Verification items for the finished model (mm, model axes). A direction names the side the tool comes from. Give positions to 0.01 mm unless a question says otherwise; leave off trailing zeros. Write each loop counter-clockwise with the first axis right and the second up, starting at its lowest first coordinate (ties: lowest second). Pieces come first, ordered by that corner, then holes.
from build123d import *

# Parameters (mm, degrees)
F1_DEPTH     = 20
F2_T1_DEPTH  = 20
F2_T3_DEPTH  = 35
F3_T1_DEPTH  = 4
F3_T3_DEPTH  = 23.5
F3_T5_DEPTH  = 38.5
F3_T8_ANGLE  = 89.9999999987
F3_T10_ANGLE = 89.9999999987
F3_T12_ANGLE = 89.9999999987
F3_T14_ANGLE = 89.9999999987
F3_T18_ANGLE = 359.64
F3_S19_R     = 5
F3_T20_DEPTH = 6
F3_T24_ANGLE = 359.64
F3_S25_R     = 5
F3_T26_DEPTH = 6
F3_T30_ANGLE = 328.8283154119
F3_S31_R     = 5
F3_T32_DEPTH = 6
F3_T36_ANGLE = 328.8283154119
F3_S37_R     = 5
F3_T38_DEPTH = 6


# Not quite as in the source:
# - a fillet or chamfer that OpenCascade refuses, or shapes differently, is made with other operations: its cross-section is extruded or revolved along the edge and cut away or added


with BuildPart() as f1:
    # F0 (on Right) → F1 (new body)
    with BuildSketch(Plane.YZ):
        Polygon((0, -10.05617938), (0, 24.94382062), (-3, 24.94382062), (-3, -7.05617938), (-13, -7.05617938), (-13, 9.94382062), (-16, 9.94382062), (-16, -10.05617938), align=None)
    extrude(amount=F1_DEPTH)

    # F2: fillet of radius 3 on 5 edges, made by hand

    # F2_s2 → F2_t1 (join)
    with BuildSketch(Plane.YZ):
        with BuildLine():
            ThreePointArc((-10, -7.05617938), (-12.1213203436, -6.1774997235), (-13, -4.05617938))
            Line((-13, -4.05617938), (-13, -7.05617938))
            Line((-13, -7.05617938), (-10, -7.05617938))
        make_face()
        with BuildLine():
            ThreePointArc((-3, -4.05617938), (-3.8786796564, -6.1774997235), (-6, -7.05617938))
            Line((-6, -7.05617938), (-3, -7.05617938))
            Line((-3, -7.05617938), (-3, -4.05617938))
        make_face()
    extrude(amount=F2_T1_DEPTH)

    # F2_s4 → F2_t3 (cut)
    with BuildSketch(Plane.YZ.offset(-7.5)):
        with BuildLine():
            ThreePointArc((0, 24.94382062), (-2.1213203436, 24.0651409636), (-3, 21.94382062))
            Line((-3, 21.94382062), (-3, 24.94382062))
            Line((-3, 24.94382062), (0, 24.94382062))
        make_face()
        with BuildLine():
            ThreePointArc((-13, 6.94382062), (-13.8786796564, 9.0651409636), (-16, 9.94382062))
            Line((-16, 9.94382062), (-13, 9.94382062))
            Line((-13, 9.94382062), (-13, 6.94382062))
        make_face()
        with BuildLine():
            ThreePointArc((-16, 6.94382062), (-15.1213203436, 9.0651409636), (-13, 9.94382062))
            Line((-13, 9.94382062), (-16, 9.94382062))
            Line((-16, 9.94382062), (-16, 6.94382062))
        make_face()
    extrude(amount=F2_T3_DEPTH, mode=Mode.SUBTRACT)

    # F3: fillet of radius 5 on 4 edges, made by hand

    # F3_s2 → F3_t1 (cut)
    with BuildSketch(Plane.XZ.offset(6)):
        with BuildLine():
            ThreePointArc((20, -12.05617938), (18.5355339059, -8.520645474), (15, -7.05617938))
            Line((15, -7.05617938), (20, -7.05617938))
            Line((20, -7.05617938), (20, -12.05617938))
        make_face()
        with BuildLine():
            ThreePointArc((0, -12.05617938), (1.4644660941, -8.520645474), (5, -7.05617938))
            Line((5, -7.05617938), (0, -7.05617938))
            Line((0, -7.05617938), (0, -12.05617938))
        make_face()
    extrude(amount=F3_T1_DEPTH, mode=Mode.SUBTRACT)

    # F3_s4 → F3_t3 (cut)
    with BuildSketch(Plane.XY.offset(-4.05617938)):
        with BuildLine():
            ThreePointArc((20, -18), (18.5355339059, -14.4644660941), (15, -13))
            Line((15, -13), (20, -13))
            Line((20, -13), (20, -18))
        make_face()
        with BuildLine():
            ThreePointArc((0, -18), (1.4644660941, -14.4644660941), (5, -13))
            Line((5, -13), (0, -13))
            Line((0, -13), (0, -18))
        make_face()
    extrude(amount=F3_T3_DEPTH, mode=Mode.SUBTRACT)

    # F3_s6 → F3_t5 (cut)
    with BuildSketch(Plane.XY.offset(-4.05617938)):
        with BuildLine():
            ThreePointArc((20, 2), (18.5355339059, -1.5355339059), (15, -3))
            Line((15, -3), (20, -3))
            Line((20, -3), (20, 2))
        make_face()
        with BuildLine():
            ThreePointArc((0, 2), (1.4644660941, -1.5355339059), (5, -3))
            Line((5, -3), (0, -3))
            Line((0, -3), (0, 2))
        make_face()
    extrude(amount=F3_T5_DEPTH, mode=Mode.SUBTRACT)

    # F3_s7 → F3_t8 (revolve, cut)
    with BuildSketch(Plane.XY.offset(-4.05617938)):
        with BuildLine():
            ThreePointArc((0, 2), (1.4644660941, -1.5355339059), (5, -3))
            Line((5, -3), (0, -3))
            Line((0, -3), (0, 2))
        make_face()
    revolve(axis=Axis((0, -6, -4.05617938), (-1, 0, 0)), revolution_arc=F3_T8_ANGLE, mode=Mode.SUBTRACT)

    # F3_s9 → F3_t10 (revolve, cut)
    with BuildSketch(Plane.XY.offset(-4.05617938)):
        with BuildLine():
            ThreePointArc((20, 2), (18.5355339059, -1.5355339059), (15, -3))
            Line((15, -3), (20, -3))
            Line((20, -3), (20, 2))
        make_face()
    revolve(axis=Axis((20, -6, -4.05617938), (-1, 0, 0)), revolution_arc=F3_T10_ANGLE, mode=Mode.SUBTRACT)

    # F3_s11 → F3_t12 (revolve, cut)
    with BuildSketch(Plane.XZ.offset(10)):
        with BuildLine():
            ThreePointArc((0, -12.05617938), (1.4644660941, -8.5206454741), (5, -7.05617938))
            Line((5, -7.05617938), (0, -7.05617938))
            Line((0, -7.05617938), (0, -12.05617938))
        make_face()
    revolve(axis=Axis((0, -10, -4.05617938), (-1, 0, 0)), revolution_arc=F3_T12_ANGLE, mode=Mode.SUBTRACT)

    # F3_s13 → F3_t14 (revolve, cut)
    with BuildSketch(Plane.XZ.offset(10)):
        with BuildLine():
            ThreePointArc((20, -12.05617938), (18.5355339059, -8.5206454741), (15, -7.05617938))
            Line((15, -7.05617938), (20, -7.05617938))
            Line((20, -7.05617938), (20, -12.05617938))
        make_face()
    revolve(axis=Axis((20, -10, -4.05617938), (-1, 0, 0)), revolution_arc=F3_T14_ANGLE, mode=Mode.SUBTRACT)


with BuildPart() as f3_tool16:
    # F3_s17 → F3_t18 (revolve)
    with BuildSketch(Plane(origin=(0, 0.0429965174, 6.8430181729), x_dir=(1, 0, 0), z_dir=(0, 0.006283144, 0.9999802609))):
        with BuildLine():
            ThreePointArc((19.5825756949, -16.0433131985), (17.7386127875, -13.8600130659), (15, -13.0433131986))
            Line((15, -13.0433131986), (20, -13.0433131986))
            Line((20, -13.0433131986), (20, -16.0433131985))
            Line((20, -16.0433131985), (19.5825756949, -16.0433131985))
        make_face()
    revolve(axis=Axis((20, -15.9999999999, 6.9438206201), (-1, 0, 0)), revolution_arc=F3_T18_ANGLE)

    # F3_s19 → F3_t20 (cut, symmetric)
    with BuildSketch(Plane.XY.offset(6.9)):
        with Locations((15, -18)):
            Circle(F3_S19_R)
    extrude(amount=F3_T20_DEPTH, both=True, mode=Mode.SUBTRACT)


with BuildPart() as f1_1:
    add(f1.part)

    # F3_t15: cut F3_tool16
    add(f3_tool16.part, mode=Mode.SUBTRACT)


with BuildPart() as f3_tool22:
    # F3_s23 → F3_t24 (revolve)
    with BuildSketch(Plane(origin=(0, 0.0429965174, 6.8430181729), x_dir=(1, 0, 0), z_dir=(0, 0.006283144, 0.9999802609))):
        with BuildLine():
            ThreePointArc((0.4174243051, -16.0433131985), (2.2613872125, -13.8600130659), (5, -13.0433131986))
            Line((5, -13.0433131986), (0, -13.0433131986))
            Line((0, -13.0433131986), (0, -16.0433131985))
            Line((0, -16.0433131985), (0.4174243051, -16.0433131985))
        make_face()
    revolve(axis=Axis((0, -15.9999999999, 6.9438206201), (-1, 0, 0)), revolution_arc=F3_T24_ANGLE)

    # F3_s25 → F3_t26 (cut, symmetric)
    with BuildSketch(Plane.XY.offset(6.9)):
        with Locations((5, -18)):
            Circle(F3_S25_R)
    extrude(amount=F3_T26_DEPTH, both=True, mode=Mode.SUBTRACT)


with BuildPart() as f1_2:
    add(f1_1.part)

    # F3_t21: cut F3_tool22
    add(f3_tool22.part, mode=Mode.SUBTRACT)


with BuildPart() as f3_tool28:
    # F3_s29 → F3_t30 (revolve)
    with BuildSketch(Plane.XY.offset(21.9438206201)):
        with BuildLine():
            ThreePointArc((15, -3), (17.7386127875, -2.1833001327), (19.5825756949, -1e-10))
            Line((19.5825756949, -1e-10), (20, -1e-10))
            Line((20, -1e-10), (20, -3))
            Line((20, -3), (15, -3))
        make_face()
    revolve(axis=Axis((20, -1e-10, 21.9438206201), (-1, 0, 0)), revolution_arc=F3_T30_ANGLE)

    # F3_s31 → F3_t32 (cut, symmetric)
    with BuildSketch(Plane.XY.offset(21.9)):
        with Locations((15, 2)):
            Circle(F3_S31_R)
    extrude(amount=F3_T32_DEPTH, both=True, mode=Mode.SUBTRACT)


with BuildPart() as f1_3:
    add(f1_2.part)

    # F3_t27: cut F3_tool28
    add(f3_tool28.part, mode=Mode.SUBTRACT)


with BuildPart() as f3_tool34:
    # F3_s35 → F3_t36 (revolve)
    with BuildSketch(Plane.XY.offset(21.9438206201)):
        with BuildLine():
            ThreePointArc((5, -3), (2.2613872125, -2.1833001327), (0.4174243051, -1e-10))
            Line((0.4174243051, -1e-10), (0, -1e-10))
            Line((0, -1e-10), (0, -3))
            Line((0, -3), (5, -3))
        make_face()
    revolve(axis=Axis((0, -1e-10, 21.9438206201), (-1, 0, 0)), revolution_arc=F3_T36_ANGLE)

    # F3_s37 → F3_t38 (cut, symmetric)
    with BuildSketch(Plane.XY.offset(21.9)):
        with Locations((5, 2)):
            Circle(F3_S37_R)
    extrude(amount=F3_T38_DEPTH, both=True, mode=Mode.SUBTRACT)


with BuildPart() as f1_4:
    add(f1_3.part)

    # F3_t33: cut F3_tool34
    add(f3_tool34.part, mode=Mode.SUBTRACT)


solid = f1_4.part
Item 1: Sectioned sample at B-B on x = 10.25. Record the cut outline in (y, z), then the cut area to 3 significant figures.
Answer key:
outline: (-16, -10.06) - (0, -10.06) - (0, 24.94) arc R3 ccw to (-3, 21.94) - (-3, -4.06) arc R3 cw to (-6, -7.06) - (-10, -7.06) arc R3 cw to (-13, -4.06) - (-13, 6.94) arc R3 ccw to (-14.5, 9.54) arc R3 ccw to (-16, 6.94) - close
area: 193 mm2
Item 2: Set-up check for faces 1 (the face through (9.9, -3.9, -6.2)), 2 (the face through (2.228, -7.972, -7.895)), 3 (the face through (18, -2, 10)): record each of +Z, -Z, +X, -X, +Y, -Y from which the full face is reachable in a straight line by a thin tool's end or side.
Answer key:
face 1: +Z, +X, -X
face 2: +Z, -X
face 3: +Z, +X
Item 3: Sectioned sample at D-D on y = -7.25. Record the cut outline in (x, z).
Answer key:
outline: (0.42, -10.06) - (19.58, -10.06) arc R5 ccw to (15, -7.06) - (5, -7.06) arc R5 ccw to start
Item 4: Scan lines: line 1 along Y through (x, z) = (9.25, 17); line 2 along Y through (x, z) = (5, 6.5); line 3 along Y through (x, z) = (15.5, -6.5). Record each from-to range of solid material in increasing order.
Answer key:
line 1: y = -3 to 0
line 2: y = -16 to -13, -3 to 0
line 3: y = -16 to -11.78, -4.22 to 0
Item 5: Sectioned sample at A-A on z = 4. Record the cut outline in (x, y), then the cut area to 3 significant figures.
Answer key:
outline: (0.42, -16) - (19.58, -16) arc R5 ccw to (15, -13) - (5, -13) arc R5 ccw to start; (0.42, 0) arc R5 ccw to (5, -3) - (15, -3) arc R5 ccw to (19.58, 0) - close
area: 99.6 mm2
Item 6: Sectioned sample at C-C on z = 8. Record the cut outline in (x, y), then the cut area to 3 significant figures.
Answer key:
outline: (0.42, 0) arc R5 ccw to (5, -3) - (15, -3) arc R5 ccw to (19.58, 0) - close; (0.51, -15.81) - (19.49, -15.81) arc R5 ccw to (16.37, -13.19) - (3.63, -13.19) arc R5 ccw to start
area: 93.7 mm2
Item 7: Release check for a two-part mould opening along Y. For faces 4 (the face through (10, 0, 7)), 5 (the face through (18, -14, 3)), 6 (the face through (10, -16, -1)), 7 (the face through (2, -14, 3)) record: released by +Y, released by -Y, zero draft, split by the parting line, or undercut.
Answer key:
face 4: released by +Y
face 5: undercut
face 6: released by -Y
face 7: undercut
Item 8: Depth check by flat-ended pin: pin 1 (3 mm diameter, centred on x = 11, y = -7.5, fed in from +Z); pin 2 (6 mm diameter, centred on x = 4, z = 18, fed in from -Y). Enter the tip coordinate at first touch or a pass-through.
Answer key:
pin 1: stops at z = -7.06
pin 2: stops at y = -3
